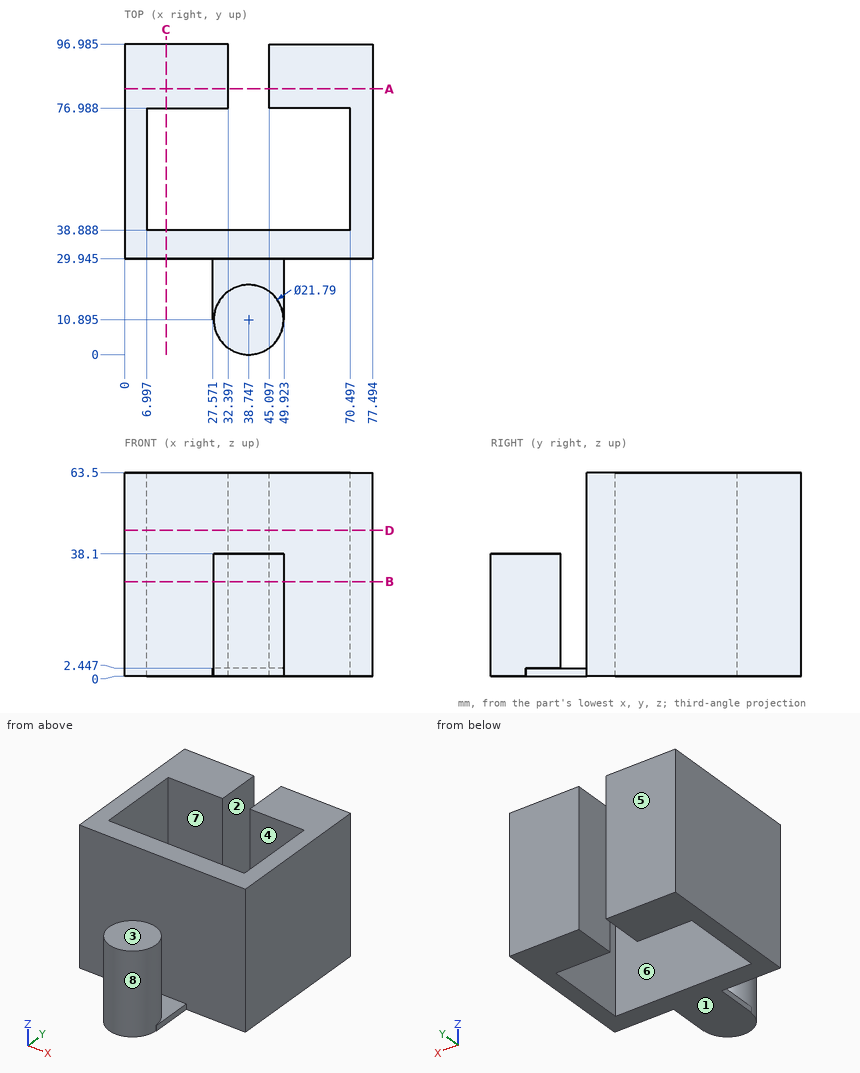
The drawing under review shows one solid part. Ordinate dimensions are in mm from its lowest x, y, z. A direction names the side the tool comes from. Round coordinates to 2 decimals unless told otherwise and drop trailing zeros. Order: outer loops, then holes, each group sorted by start corner. A loop starts at its lowest first (then second) coordinate and runs counter-clockwise, first axis right, second up. Notation, with made-up numbers: (-35.75, 3) -> (-9.75, 3) arc R15 ccw to (-9.75, 31) -> close; hole circle Ø9 at (81.5, -7). An arc over 180 degrees is marked (long way). Return JSON: item names as keys, results as strings.
1. Take a section at A-A (y = 83). Write out the cut boundary in (x, z) (1 decimal).
Answer block:
{"outline": "(0, 0) -> (32.4, 0) -> (32.4, 63.5) -> (0, 63.5) -> close; (45.1, 0) -> (77.5, 0) -> (77.5, 63.5) -> (45.1, 63.5) -> close"}
2. Take a section at B-B (z = 29.5). Write out the cut boundary in (x, y) (1 decimal).
Answer block:
{"outline": "(0, 29.9) -> (77.5, 29.9) -> (77.5, 97) -> (45.1, 97) -> (45.1, 77) -> (70.5, 77) -> (70.5, 38.9) -> (7, 38.9) -> (7, 77) -> (32.4, 77) -> (32.4, 97) -> (0, 97) -> close; circle Ø21.8 at (38.7, 10.9)"}
3. For the marked faces 1, 2, 3 and 4, list the 3-axis set-ups (+Z, -Z, +X, -X, +Y, -Y) from which the entire face can be reached by the end or side of a thin tool; tool diameter is ignored.
Answer block:
{"face 1": "-Z, +X, -X, +Y, -Y", "face 2": "+Z, -Z, +Y", "face 3": "+Z, +X, -X, -Y", "face 4": "+Z, -Z"}
4. Insertion check: P1, Ø1.2, axis at y = 20, z = 1, coming from the +X side; P2, Ø10, axis at x = 63.5, z = 20.5, coming from the -Y side (1 decimal); P3, Ø17.5, axis at x = 37.5, y = 8.5, coming from the +Z side. Each pin has a flat end and moves straight along its axis. Give the tip position at first contact, or say it passes through.
Answer block:
{"P1": "stops at x = 49.92", "P2": "stops at y = 29.9", "P3": "stops at z = 38.1"}
5. For L1, parallel to Y at x = 23, z = 37 (1 decimal); L2, parallel to X at y = 74.5, z = 49 (1 decimal); L3, parallel to Y at x = 31, z = 11 (1 decimal), list the stretches that pass through material, from the lowest coordinate up. Write a range as [from, to].
Answer block:
{"L1": "y = [29.9, 38.9], [77, 97]", "L2": "x = [0, 7], [70.5, 77.5]", "L3": "y = [3.2, 18.6], [29.9, 38.9], [77, 97]"}
6. Take a section at C-C (x = 13). Write out the cut boundary in (y, z) (1 decimal).
Answer block:
{"outline": "(29.9, 0) -> (38.9, 0) -> (38.9, 63.5) -> (29.9, 63.5) -> close; (77, 0) -> (97, 0) -> (97, 63.5) -> (77, 63.5) -> close"}
7. The part is to be moulded in two halves that separate along X. For the marked faces 5, 6, 7 and 8, say which applies: +X half, -X half, draft (parallel to the pull), parting line (faces both ways), or undercut.
Answer block:
{"face 5": "draft", "face 6": "undercut", "face 7": "undercut", "face 8": "parting line"}
8. Take a section at D-D (z = 45.5). Write out the cut boundary in (x, y) (1 decimal).
Answer block:
{"outline": "(0, 29.9) -> (77.5, 29.9) -> (77.5, 97) -> (45.1, 97) -> (45.1, 77) -> (70.5, 77) -> (70.5, 38.9) -> (7, 38.9) -> (7, 77) -> (32.4, 77) -> (32.4, 97) -> (0, 97) -> close"}
